Model file for the job. Use its own axes, mm. Give positions to 0.01 mm unless a question says otherwise; leave off trailing zeros. Order: outer loops, then holes, each group sorted by start corner. A loop starts at its lowest first (then second) coordinate and runs counter-clockwise, first axis right, second up. Notation, with made-up numbers: M 13,51 L 48,51 A26 cw 48,74 Z; hole C -26.5,6.25 d11. An arc over 180 degrees is marked long. Return JSON: item names as keys, results as strings. Group by question number.
1. Pin check, flat tips, straight feed: pin 1 (6 mm diameter, centred on x = 6, z = 0, fed in from +Y); pin 2 (1 mm diameter, centred on x = -1, y = -53.5, fed in from +Z); pin 3 (3 mm diameter, centred on x = 0.5, z = -0.5, fed in from -Y); pin 4 (1 mm diameter, centred on y = -9, z = 5.5, fed in from -X). Stop position of each tip, or through.
2. Wall check: probe 1 along X at (y, z) = (-7, -0.25); probe 2 along X at (y, z) = (-67, -5.5); probe 3 along Y at (x, z) = (4.25, 6). Give the ranges that are in metal, low to high. Write a range as [from, to].
3. Two-plate mould, pull along Y, no slides. Class faces 1 (the face through (0, 0, 0)), 2 (the face through (-1.172, -34.51, 8.923)), 3 (the face through (-1, -67.727, -7)), 4 (the face through (5, -70, -6)): released by +Y, released by -Y, zero draft, split by the parting line, or undercut.
4. Slice it at A-A on y = -10.5. List the corners of the cut face in (x, z).
from build123d import *

# Parameters (mm, degrees)
F0_R     = 9
F1_DEPTH = 70


with BuildPart() as f1:
    # F0 (on Front) → F1 (new body)
    with BuildSketch(Plane.XZ):
        Circle(F0_R)
    extrude(amount=F1_DEPTH)

    # F2 (on Right) → F3 (revolve, cut)
    with BuildSketch(Plane.YZ):
        with BuildLine():
            Line((-65.6930357218, -6.7071020603), (-65.6930357218, -7.2155290418))
            add(Edge.make_bspline(
                [(-65.6930357218, -7.2155290418), (-54.8685416579, -5.6061186379), (-54.8685416579, 0)],
                knots=[5.0035671981, 5.0035671981, 5.0035671981, 6.2831853072, 6.2831853072, 6.2831853072], degree=2, weights=[1, 0.802209775, 1]))
            Line((-54.8685416579, 0), (-65.6930357218, 0))
            Line((-65.6930357218, 0), (-67.727163434, 0))
            Line((-67.727163434, 0), (-70.0518861413, 0))
            Line((-70.0518861413, 0), (-70.0518861413, -7.5326042516))
            Line((-70.0518861413, -7.5326042516), (-67.727163434, -6.7071020603))
            Line((-67.727163434, -6.7071020603), (-67.727163434, -7.443788395))
            Line((-67.727163434, -7.443788395), (-65.6930357218, -6.7071020603))
        make_face()
    revolve(axis=Axis((0, -60.2807886899, 0), (0, 1, 0)), mode=Mode.SUBTRACT)


solid = f1.part
Result:
{
 "1": {"pin 1": "stops at y = 0", "pin 2": "stops at z = 8.99", "pin 3": "stops at y = -55.53", "pin 4": "stops at x = -7.48"},
 "2": {"probe 1": "x = [-9, 9]", "probe 2": "x = [-7.12, -4.62], [4.62, 7.12]", "probe 3": "y = [-69.55, -67.73], [-67.48, 0]"},
 "3": {"face 1": "released by +Y", "face 2": "zero draft", "face 3": "undercut", "face 4": "released by -Y"},
 "4": {"outline": "C 0,0 d18"}
}
